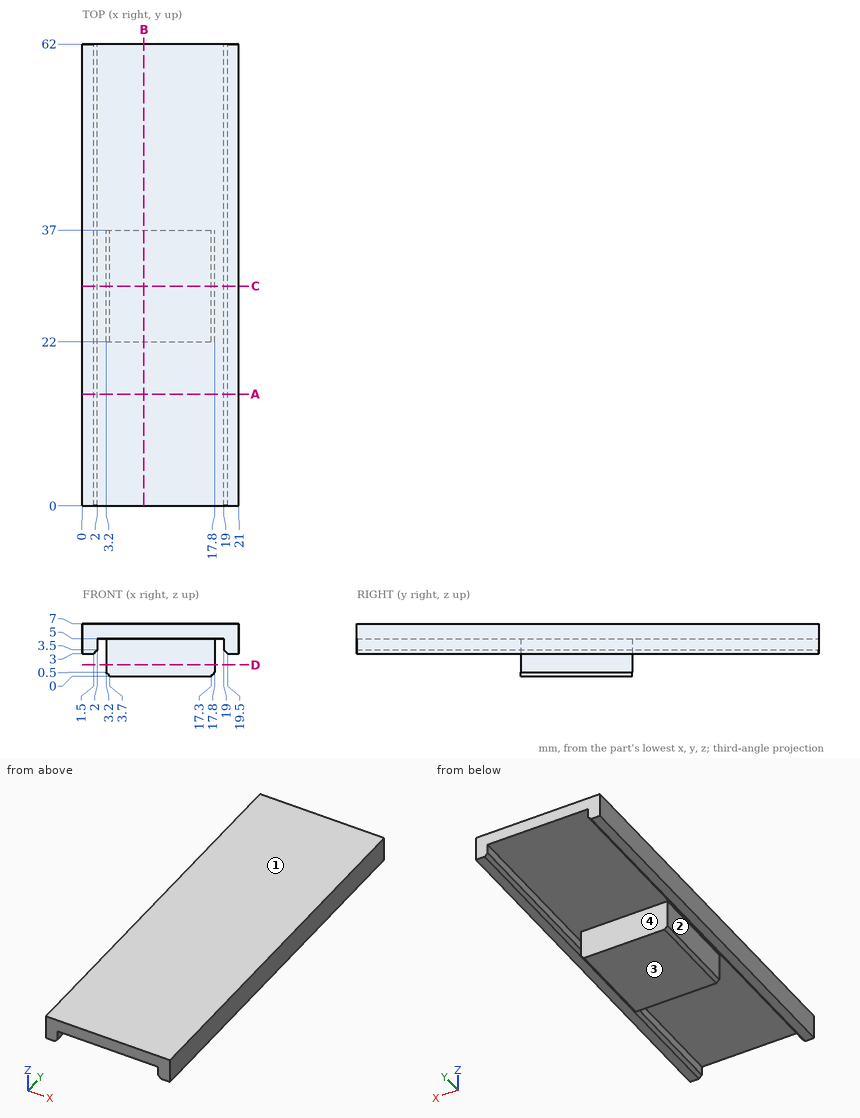
Here's the drawing with two shaded views (mm, measured from the low corner). I have some questions. A direction names the side the tool comes from. Round coordinates to 2 decimals unless told otherwise and drop trailing zeros. Write each loop counter-clockwise with the first axis right and the second up, starting at its lowest first coordinate (ties: lowest second). Pieces come first, ordered by that corner, then holes. Notation, with made-up numbers: M 6,-14 L 37,-14 A22 ccw 37,22 Z; hole C 28,10 d2. An arc over 180 degrees is marked long. Use CSV: the item, a comma, the result in double quotes.
(1) Imagine slicing it at C-C (y = 29.5). Write out the boundary of the cut face in (x, z), plus the area to 4 significant figures.
Check values:
outline,"M 0,3 L 1.5,3 L 2,3.5 L 2,5 L 3.2,5 L 3.2,0.5 L 3.7,0 L 17.3,0 L 17.8,0.5 L 17.8,5 L 19,5 L 19,3.5 L 19.5,3 L 21,3 L 21,7 L 0,7 Z"
area,"122.5 mm^2"
(2) I need wall thicknesses on line 1 along X through (y, z) = (42, 4.75); line 2 along X through (y, z) = (36, 1.5); line 3 along Z through (x, y) = (4.75, 5.5). Which ranges of each line are inside material? Lowest first, please.
Check values:
line 1,"0 to 2, 19 to 21"
line 2,"3.2 to 17.8"
line 3,"5 to 7"
(3) I'm going to push flat-ended pins straight in: pin 1 (1.6 mm diameter, centred on x = 20, y = 33.5, fed in from -Z); pin 2 (3 mm diameter, centred on x = 9, z = 3, fed in from -Y); pin 3 (1 mm diameter, centred on x = 7.5, y = 8, fed in from -Z). Where does each tip first touch, or does it pass through?
Check values:
pin 1,"z = 3"
pin 2,"y = 22"
pin 3,"z = 5"
(4) Imagine slicing it at D-D (z = 1.5). Write out the boundary of the cut face in (x, y), plus the area to 3 significant figures.
Check values:
outline,"M 3.2,22 L 17.8,22 L 17.8,37 L 3.2,37 Z"
area,"219 mm^2"
(5) On a 3-axis mill with a long thin cutter (end or side, diameter ignored), from which of +Z, -Z, +X, -X, +Y, -Y can I reach the whole of each face in a straight line? I mean the marked faces 1 and 2. Say none if no direction works.
Check values:
face 1,"+Z, +X, -X, +Y, -Y"
face 2,"-Z, +Y, -Y"
(6) Imagine slicing it at B-B (x = 8.25). Write out the boundary of the cut face in (y, z), plus the area to 3 significant figures.
Check values:
outline,"M 0,5 L 22,5 L 22,0 L 37,0 L 37,5 L 62,5 L 62,7 L 0,7 Z"
area,"199 mm^2"
(7) Imagine slicing it at A-A (y = 15). Write out the boundary of the cut face in (x, z), plus the area to 4 significant figures.
Check values:
outline,"M 0,3 L 1.5,3 L 2,3.5 L 2,5 L 19,5 L 19,3.5 L 19.5,3 L 21,3 L 21,7 L 0,7 Z"
area,"49.75 mm^2"
(8) We'd pull the mould along X, two halves only. Please class the marked faces 3 and 4: +X half, -X half, draft (parallel to the pull), parting line (faces both ways), or undercut.
Check values:
face 3,"draft"
face 4,"undercut"
